The model under review builds one solid part; all positions refer to its coordinate system, in mm. A direction names the side the tool comes from. Round coordinates to 2 decimals unless told otherwise and drop trailing zeros. Order: outer loops, then holes, each group sorted by start corner. A loop starts at its lowest first (then second) coordinate and runs counter-clockwise, first axis right, second up. Notation, with made-up numbers: (-14, 29.5) -> (-5, 29.5) arc R23 ccw to (-5, 58.5) -> close; hole circle Ø2 at (57.25, 43). An arc over 180 degrees is marked (long way). Return JSON: item names as keys, results as strings. Group by question number.
Autodesk Inventor part; units mm, degrees
ref_plane "YZ Plane" through (0, 0, 0) normal (1, 0, 0) x (0, 1, 0)
ref_plane "XZ Plane" through (0, 0, 0) normal (0, 1, 0) x (-1, 0, 0)
ref_plane "XY Plane" through (0, 0, 0) normal (0, 0, 1) x (1, 0, 0)
sketch "Sketch1" plane through (0, 0, 0) normal (1, 0, 0) x (0, 1, 0)
  line L0 (32.6613, 26.3105) -> (-7.3387, 26.3105)
  line L1 (-7.3387, 26.3105) -> (-7.3387, -27.6895)
  line L2 (-7.3387, -27.6895) -> (32.6613, -27.6895)
  line L3 (32.6613, -27.6895) -> (32.6613, 26.3105)
  point P0 (0, 0)
  dimension "d0" = 40
  dimension "d1" = 54
extrude "Extrusion1" add sketch "Sketch1" along normal blind 5
sketch "Sketch2" plane through (0, -7.3387, 26.3105) normal (0, 0, 1) x (1, 0, 0)
  line L0 (5, 0) -> (-20, 0)
  line L1 (-20, 0) -> (-20, -5)
  line L2 (-20, -5) -> (5, -5)
  line L3 (5, -5) -> (5, 0)
  point P0 (0, 7.3387)
  dimension "d4" = 5
  dimension "d5" = 25
extrude "Extrusion2" add sketch "Sketch2" against normal blind 54
sketch "Sketch3" plane through (5, 0, 0) normal (1, 0, 0) x (0, 0, -1)
  line L0 (-26.3105, 32.6613) -> (-26.3105, -12.3387)
  line L1 (-26.3105, -12.3387) -> (-14.3105, -12.3387)
  line L2 (-14.3105, -12.3387) -> (-14.3105, 2.6613)
  line L3 (-14.3105, 2.6613) -> (-26.3105, 2.6613)
  line L4 (-26.3105, 2.6613) -> (-26.3105, -12.3387)
  line L5 (-26.3105, -12.3387) -> (27.6895, -12.3387)
  line L6 (27.6895, -12.3387) -> (15.6895, -12.3387)
  line L7 (15.6895, -12.3387) -> (15.6895, 2.6613)
  line L8 (15.6895, 2.6613) -> (27.6895, 2.6613)
  line L9 (27.6895, 2.6613) -> (27.6895, -12.3387)
  point P0 (0, 0)
  point P1 (15.6895, -12.3387)
  dimension "d8" = 12
  dimension "d9" = 12
  dimension "d10" = 15
  dimension "d11" = 15
extrude "Extrusion3" cut sketch "Sketch3" against normal through all
fillet "Fillet1" radius 2 4 edges at (2.5, 2.6613, 26.3105) (2.5, 2.6613, -27.6895) (2.5, 32.6613, -27.6895) (2.5, 32.6613, 26.3105)
fillet "Fillet2" radius 2 1 edges at (0, -7.3387, -0.6895)
sketch "Sketch4" plane through (-20, -7.3387, 14.3105) normal (0, 1, 0) x (1, 0, 0)
  arc A0 (10.7679, 21.3) -> (4.5679, 21.3) centre (7.6679, 21.3) ccw
  arc A1 (4.5679, 8.9679) -> (10.7679, 8.9679) centre (7.6679, 8.9679) ccw
  line L0 (10.7679, 21.3) -> (10.7679, 8.9679)
  line L1 (4.5679, 21.3) -> (4.5679, 8.9679)
  line L2 (18, 30) -> (0, 30)
  point P0 (20, 14.3105)
  dimension "d16" = 6.2
  dimension "d17" = 6.2
  dimension "d18" = 8.7
extrude "Extrusion4" cut sketch "Sketch4" against normal through all
fillet "Fillet3" radius 2 1 edges at (5, -12.3387, -0.6895)
properties part number "end plate"
Item 1: Consider section C-C on y = 22. State the section outline as (x, z) points.
Item 2: Consider section A-A on z = -2.5. State the section outline as (x, y) points, plus the area to 3 significant figures.
Item 3: The part is to be moulded in two halves that separate along X. For faces 1 (the face through (-12.4, -9.8, 8.44)), 2 (the face through (-20, -10, 0)), 3 (the face through (-12.26, -9.8, -10.09)), 4 (the face through (3, 2.661, -21)), say which applies: +X half, -X half, draft (parallel to the pull), parting line (faces both ways), or undercut.
Item 4: Wall thickness on line 1 along X through (y, z) = (-10, 3); line 2 along Y through (x, z) = (-13.5, 9); line 3 along Y through (x, z) = (2.5, 20.5): over which ranges is each line inside the solid? List them lowest first.
Item 5: Consider section D-D on x = -7.75. State the section outline as (y, z) points.
Item 6: Insertion check: pin 1 Ø9 at (x, z) = (-10.5, -2) entering from +Y; pin 2 Ø11.5 at (y, z) = (20.5, 0) entering from -X; pin 3 Ø6 at (x, y) = (-2, -3.5) entering from +Z. Each pin has a flat end and moves straight along its axis. Give the tip position at first contact, or say it passes through.
Item 7: For faces 5 (the face through (-9.232, -10, -1)), 6 (the face through (0, 13, 0)), 7 (the face through (-5, -8, 14.31)), 8 (the face through (-5, -8, -15.69)), list the 3-axis set-ups (+Z, -Z, +X, -X, +Y, -Y) from which the entire face can be reached by the end or side of a thin tool; tool diameter is ignored.
Item 8: Consider section B-B on x = -11.5. State the section outline as (y, z) points, plus the area to 3 significant figures.
Values:
{
 "1": {"outline": "(0, -27.69) -> (5, -27.69) -> (5, 26.31) -> (0, 26.31) -> close"},
 "2": {"outline": "(-20, -12.34) -> (-15.43, -12.34) -> (-15.43, -7.34) -> (-20, -7.34) -> close; (-9.23, -12.34) -> (3, -12.34) arc R2 ccw to (5, -10.34) -> (5, 32.66) -> (0, 32.66) -> (0, -5.34) arc R2 cw to (-2, -7.34) -> (-9.23, -7.34) -> close", "area": "294 mm^2"},
 "3": {"face 1": "undercut", "face 2": "-X half", "face 3": "undercut", "face 4": "draft"},
 "4": {"line 1": "-20 to -15.43, -9.23 to 5", "line 2": "-12.34 to -7.34", "line 3": "2.66 to 32.66"},
 "5": {"outline": "(-12.34, -15.69) -> (-7.34, -15.69) -> (-7.34, 14.31) -> (-12.34, 14.31) -> close"},
 "6": {"pin 1": "y = -7.34", "pin 2": "x = 0", "pin 3": "z = 14.31"},
 "7": {"face 5": "+Y, -Y", "face 6": "+Z, -Z, -X, +Y", "face 7": "+Z, +X, -X, -Y", "face 8": "-Z, +X, -X, -Y"},
 "8": {"outline": "(-12.34, -15.69) -> (-7.34, -15.69) -> (-7.34, -9.98) -> (-12.34, -9.98) -> close; (-12.34, 8.33) -> (-7.34, 8.33) -> (-7.34, 14.31) -> (-12.34, 14.31) -> close", "area": "58.5 mm^2"}
}
